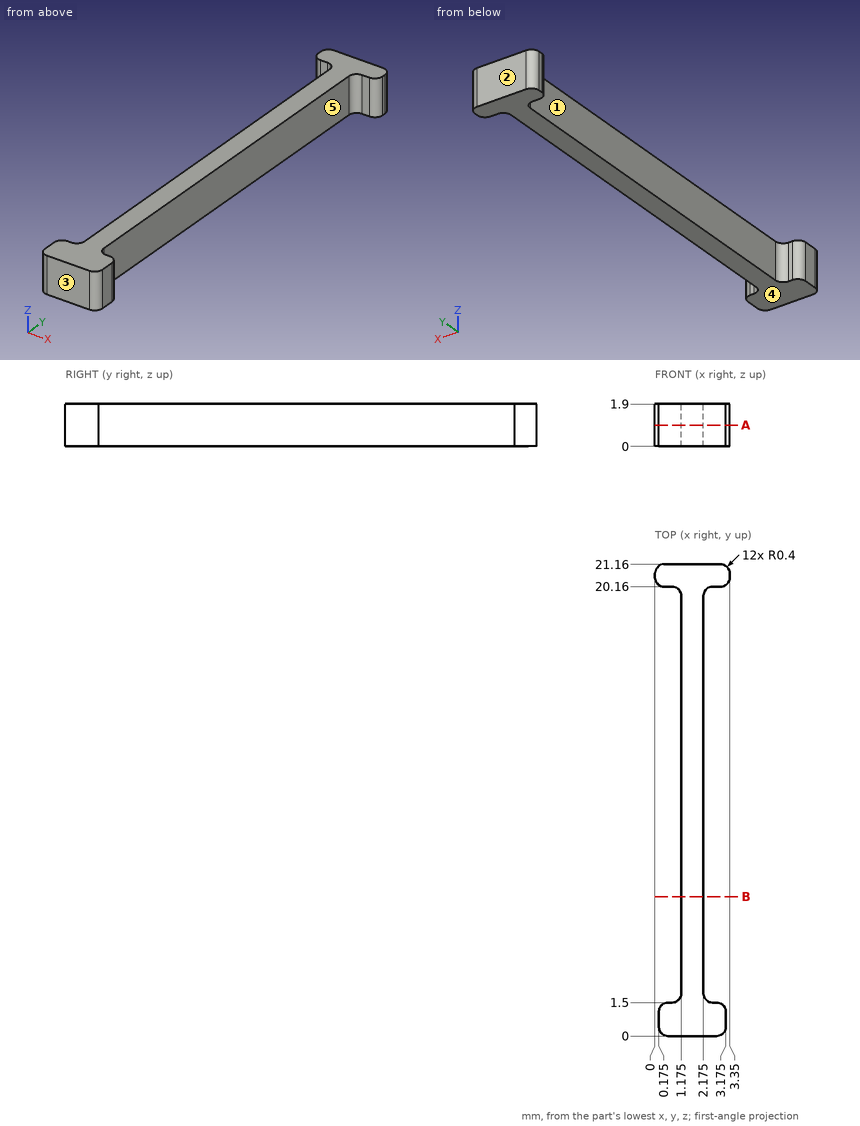
Part print with two shaded views. Sizes in mm from the minimum x, y, z corner. A direction names the side the tool comes from. Round coordinates to 2 decimals unless told otherwise and drop trailing zeros. Order: outer loops, then holes, each group sorted by start corner. A loop starts at its lowest first (then second) coordinate and runs counter-clockwise, first axis right, second up. Notation, with made-up numbers: M 83.5,51.5 L 98.5,51.5 A19 ccw 98.5,64.5 Z; hole C 84.5,20 d4. An arc over 180 degrees is marked long. Put each result on its own line as item: value. Start each with the question number.
1. Drop a flat-ended pin along its axis: pin 1 (0.6 mm diameter, centred on y = 14.5, z = 1, fed in from +X) (3 decimals). Give the stop position or say it passes through.
2. Slice it at B-B on y = 6.25. List the corners of the cut face in (x, z) (3 decimals), then the cut area to 3 significant figures.
3. Two-plate mould, pull along Y, no slides. Class the marked faces 1, 2 and 3: +Y half, -Y half, draft (parallel to the pull), parting line (faces both ways), or undercut.
4. Drill centre lines: probe 1 along Y at (x, z) = (2.7, 0.1); probe 2 along X at (y, z) = (7.75, 0.9) (3 decimals); probe 3 along Y at (x, z) = (0.3, 1.6). Where is each one in solid material? Low to high. Write a range as [from, to].
5. Slice it at A-A on z = 0.95. List the corners of the cut face in (x, y) (3 decimals).
6. Tool access for the marked faces 4 and 5: list every direction of +Z, -Z, +X, -X, +Y, -Y with a clear straight run to the whole face (end or side of a thin tool).
Findings:
1. pin 1: x = 2.175
2. outline: M 1.175,0 L 2.175,0 L 2.175,1.9 L 1.175,1.9 Z
2. area: 1.90 mm2
3. face 1: undercut
3. face 2: +Y half
3. face 3: -Y half
4. probe 1: [0, 1.5], [20.16, 21.16]
4. probe 2: [1.175, 2.175]
4. probe 3: [0.11, 1.39], [20.17, 21.15]
5. outline: M 0,20.56 A0.4 ccw 0.4,20.16 L 0.775,20.16 A0.4 cw 1.175,19.76 L 1.175,1.9 A0.4 cw 0.775,1.5 L 0.575,1.5 A0.4 ccw 0.175,1.1 L 0.175,0.4 A0.4 ccw 0.575,0 L 2.775,0 A0.4 ccw 3.175,0.4 L 3.175,1.1 A0.4 ccw 2.775,1.5 L 2.575,1.5 A0.4 cw 2.175,1.9 L 2.175,19.76 A0.4 cw 2.575,20.16 L 2.95,20.16 A0.4 ccw 3.35,20.56 L 3.35,20.76 A0.4 ccw 2.95,21.16 L 0.4,21.16 A0.4 ccw 0,20.76 Z
6. face 4: -Z, +X, -X, +Y, -Y
6. face 5: +Z, -Z, +X
